Work out the finished part from the listing and answer in its coordinate system (mm). A direction names the side the tool comes from. Coordinates: 2 decimals unless noted, no trailing zeros. Loops run counter-clockwise (first coordinate to the right, second up) from the corner with the lowest first, then second, coordinate; pieces in that order, holes last. Notation, with made-up numbers: (44.25, 31) - (100.25, 31) arc R24 cw to (100.25, 55) - close; hole circle Ø1 at (-13, -25.75). An arc over 180 degrees is marked (long way). Write each question's results on one line, items separated by ' | '. Start each with the question number.
1. Which of the six approach directions +Z, -Z, +X, -X, +Y, -Y give full straight-line access (tool end or side, diameter ignored) to faces 4 (the flat face through (-62.5, 20, 1)), 5 (the cylindrical face through (-1.264, 20.988, -94.986))?
2. A cutting plane is placed at B-B on y = 33. Determine the outline of the cut face in (x, z), then the cut area to 3 significant figures.
3. A cutting plane is placed at C-C on z = -16.5. Determine the outline of the cut face in (x, y), then the cut area to 3 significant figures.
4. Each of these flat-tipped pins is pushed along its axis until it touches: P1, Ø13, axis at x = 0, z = 40, coming from the -Y side; P2, Ø10, axis at x = 13.5, y = 43, coming from the -Z side; P3, Ø5, axis at y = 43.5, z = 56, coming from the -X side. Where does it stop, or does it pass through?
5. A cutting plane is placed at A-A on x = 0. Determine the outline of the cut face in (y, z), then the cut area to 3 significant figures.
6. Determine the mould class of faces 1 (the cylindrical face through (-1.374, 19.72, -99.985)), 2 (the cylindrical face through (1.802, 47.535, -9.277)), 3 (the cylindrical face through (59.65, 46.99, 0.52)) for opening direction X: released by +X, released by -X, zero draft, split by the parting line, or undercut.
7. Find the intervals of material crossed by line 1 along X through (y, z) = (34, -11); line 2 along Y through (x, z) = (21, -44); line 3 along X through (y, z) = (47.2, 40), in increasing order. Write a range as [from, to].
from build123d import *

# Parameters (mm, degrees)
BOSS_EXTRUDE1_DEPTH = 50
FILLET1_R           = 10
SHELL1_T            = -5
CUT_EXTRUDE2_DEPTH  = 2.5
SKETCH5_W           = 10
SKETCH5_H           = 2.5
CUT_EXTRUDE3_DEPTH  = 168.705098402
CUT_EXTRUDE4_REACH  = 130.087
SKETCH6_R           = 5
SKETCH6_R_2         = 6


with BuildPart() as part:
    # Sketch3 → Boss-Extrude1 (new body)
    with BuildSketch(Plane(origin=(0, 0, 0), x_dir=(1, 0, 0), z_dir=(0, 1, 0))):
        with BuildLine():
            Line((-62.5, -37.5), (-62.5, 37.5))
            ThreePointArc((-62.5, 37.5), (0, 100), (62.5, 37.5))
            Line((62.5, 37.5), (62.5, -37.5))
            ThreePointArc((62.5, -37.5), (0, -100), (-62.5, -37.5))
        make_face()
    extrude(amount=BOSS_EXTRUDE1_DEPTH)

    # Fillet1
    fillet1_edges = [part.edges().sort_by_distance(p)[0] for p in [
        (0, 50, 100),
        (62.5, 50, 0),
        (0, 50, -100),
        (-62.5, 50, 0),
    ]]
    fillet(fillet1_edges, radius=FILLET1_R)

    # Shell1
    shell1_openings = [part.faces().sort_by_distance(p)[0] for p in [
        (0, 0, 0),
    ]]
    offset(amount=SHELL1_T, openings=shell1_openings, kind=Kind.INTERSECTION)

    # Sketch4 → Cut-Extrude2 (cut)
    with BuildSketch(Plane.XZ):
        with BuildLine():
            Line((-60, 37.5), (-60, -37.5))
            ThreePointArc((-60, -37.5), (0, -97.5), (60, -37.5))
            Line((60, -37.5), (60, 37.5))
            ThreePointArc((60, 37.5), (0, 97.5), (-60, 37.5))
        make_face()
    extrude(amount=-CUT_EXTRUDE2_DEPTH, mode=Mode.SUBTRACT)

    # Sketch5 → Cut-Extrude3 (cut, through all)
    with BuildSketch(Plane.ZY.offset(62.5)):
        with Locations((-18.75, 1.25)):
            Rectangle(SKETCH5_W, SKETCH5_H)
        with Locations((18.75, 1.25)):
            Rectangle(SKETCH5_W, SKETCH5_H)
    extrude(amount=-CUT_EXTRUDE3_DEPTH, mode=Mode.SUBTRACT)

    # Sketch6 → Cut-Extrude4 (cut, up to next)
    with BuildSketch(Plane(origin=(0, 50, 0), x_dir=(1, 0, 0), z_dir=(0, 1, 0)), mode=Mode.PRIVATE) as cut_extrude4_sk1:
        with Locations(Location((0, 60, 0), (0, 0, 270))):
            Circle(SKETCH6_R)
    cut_extrude4_tool1 = extrude(cut_extrude4_sk1.sketch, amount=-CUT_EXTRUDE4_REACH, mode=Mode.PRIVATE) & part.part
    # Sketch6 → Cut-Extrude4 (cut, up to next)
    with BuildSketch(Plane(origin=(0, 50, 0), x_dir=(1, 0, 0), z_dir=(0, 1, 0)), mode=Mode.PRIVATE) as cut_extrude4_sk2:
        with Locations(Location((0, 15, 0), (0, 0, 270))):
            Circle(SKETCH6_R_2)
    cut_extrude4_tool2 = extrude(cut_extrude4_sk2.sketch, amount=-CUT_EXTRUDE4_REACH, mode=Mode.PRIVATE) & part.part
    # Sketch6 → Cut-Extrude4 (cut, up to next)
    with BuildSketch(Plane(origin=(0, 50, 0), x_dir=(1, 0, 0), z_dir=(0, 1, 0)), mode=Mode.PRIVATE) as cut_extrude4_sk3:
        with Locations(Location((0, -40, 0), (0, 0, 270))):
            Circle(SKETCH6_R)
    cut_extrude4_tool3 = extrude(cut_extrude4_sk3.sketch, amount=-CUT_EXTRUDE4_REACH, mode=Mode.PRIVATE) & part.part
    add(cut_extrude4_tool1.solids().sort_by_distance((0, 50, -60))[0], mode=Mode.SUBTRACT)
    add(cut_extrude4_tool2.solids().sort_by_distance((0, 50, -15))[0], mode=Mode.SUBTRACT)
    add(cut_extrude4_tool3.solids().sort_by_distance((0, 50, 40))[0], mode=Mode.SUBTRACT)


solid = part.part
Values:
1) face 4: +Z, -Z, -X, +Y, -Y | face 5: -Y
2) outline: (-62.5, -37.5) arc R62.5 ccw to (62.5, -37.5) - (62.5, 37.5) arc R62.5 ccw to (-62.5, 37.5) - close; hole (-57.5, -37.5) arc R57.5 ccw to (57.5, -37.5) - (57.5, 37.5) arc R57.5 ccw to (-57.5, 37.5) - close | area: 2,630 mm^2
3) outline: (-62.5, 2.5) - (-57.5, 2.5) - (-57.5, 40) arc R5 cw to (-52.5, 45) - (-5.81, 45) - (-5.81, 50) - (-52.5, 50) arc R10 ccw to (-62.5, 40) - close; (5.81, 45) - (52.5, 45) arc R5 cw to (57.5, 40) - (57.5, 2.5) - (62.5, 2.5) - (62.5, 40) arc R10 ccw to (52.5, 50) - (5.81, 50) - close | area: 960 mm^2
4) P1: y = 45 | P2: z = -99.32 | P3: x = -60.07
5) outline: (0, -100) - (40, -100) arc R10 ccw to (50, -90) - (50, -65) - (45, -65) - (45, -90) arc R5 cw to (40, -95) - (2.5, -95) - (2.5, -97.5) - (0, -97.5) - close; (0, 97.5) - (2.5, 97.5) - (2.5, 95) - (40, 95) arc R5 cw to (45, 90) - (45, 45) - (50, 45) - (50, 90) arc R10 ccw to (40, 100) - (0, 100) - close; (45, -55) - (50, -55) - (50, -21) - (45, -21) - close; (45, -9) - (50, -9) - (50, 35) - (45, 35) - close | area: 1,250 mm^2
6) face 1: split by the parting line | face 2: undercut | face 3: released by +X
7) line 1: [-62.5, -57.5], [57.5, 62.5] | line 2: [45, 50] | line 3: [-59.39, -5], [5, 59.39]
